Work out the finished part from the listing and answer in its coordinate system (mm). A direction names the side the tool comes from. Round coordinates to 2 decimals unless told otherwise and drop trailing zeros. Loops run counter-clockwise (first coordinate to the right, second up) from the corner with the lowest first, then second, coordinate; pieces in that order, holes last. Notation, with made-up numbers: M 36.25,63 L 44.25,63 A14 cw 44.25,88 Z; hole C 41.5,89.25 d2. An arc over 180 degrees is marked long. One line per item, written item: value.
```python
from build123d import *

# Parameters (mm, degrees)
CROQUIS1_W            = 6
CROQUIS1_H            = 15
CROQUIS2_R            = 4.41619294
CORTAR_EXTRUIR1_DEPTH = 46.572058325


with BuildPart() as part:
    # Croquis1 → Revolución1 (revolve)
    with BuildSketch(Plane.XY):
        with BuildLine():
            Line((7.75, -7.051316702), (7.433772234, -7))
            Line((7.433772234, -7), (3.25, -7))
            Line((3.25, -7), (3.25, 6))
            ThreePointArc((3.25, 6), (4.75, 7.5), (3.25, 9))
            Line((3.25, 9), (1.25, 9))
            Line((1.25, 9), (1.25, -9))
            Line((1.25, -9), (4.765255872, -9))
            Line((4.765255872, -9), (7.75, -9))
            Line((7.75, -9), (7.75, -7.051316702))
        make_face()
        Polygon((7.75, -21), (7.75, -9), (4.765255872, -9), (1.25, -9), (1.25, -21), (7.25, -21), align=None)
        with Locations((4.25, -28.5)):
            Rectangle(CROQUIS1_W, CROQUIS1_H)
    revolve(axis=Axis((-7.75, -7, 0), (0, 1, 0)))

    # Croquis2 → Cortar-Extruir1 (cut, through all)
    with BuildSketch(Plane.XY):
        with Locations((-7.75, -14.025658351)):
            Circle(CROQUIS2_R)
    extrude(amount=-CORTAR_EXTRUIR1_DEPTH, mode=Mode.SUBTRACT)


solid = part.part
```
1) Find the intervals of material crossed by probe 1 along X at (y, z) = (-22, 0); probe 2 along Z at (x, y) = (-7.75, -3); probe 3 along Y at (x, z) = (-7.75, -14), in increasing order. Write a range as from..to.
Check values:
probe 1: -22.75..-16.75, 1.25..7.25
probe 2: -11..-9, 9..11
probe 3: -36..-18.44, -9.61..-7
2) For faces 1 (the face through (-0.598, -13.928, 13.751)), 2 (the face through (-10.13, -0.41, 10.74)), 3 (the face through (-11.005, -11.041, -11.626)), determine the directions among +Z, -Z, +X, -X, +Y, -Y from which every point of the face is accessible in a straight line to the end or side of a thin tool.
Check values:
face 1: +Y, -Y
face 2: none
face 3: -Z
3) Find section A-A (z = 0). Give the vertices of the cut face in (x, y).
Check values:
outline: M -23.25,-21 L -22.75,-21 L -22.75,-36 L -16.75,-36 L -16.75,9 L -18.75,9 A1.5 ccw -18.75,6 L -18.75,-7 L -22.93,-7 L -23.25,-7.05 Z; M 1.25,-36 L 7.25,-36 L 7.25,-21 L 7.75,-21 L 7.75,-7.05 L 7.43,-7 L 3.25,-7 L 3.25,6 A1.5 ccw 3.25,9 L 1.25,9 Z
4) Find section B-B (x = -7.75). Give the vertices of the cut face in (y, z), then the cut area to 3 significant figures.
Check values:
outline: M -36,-15 L -21,-15 L -21,-15.5 L -18.44,-15.5 L -18.44,-9 L -36,-9 Z; M -36,9 L 9,9 L 9,11 A1.5 ccw 6,11 L -7,11 L -7,15.18 L -7.05,15.5 L -21,15.5 L -21,15 L -36,15 Z; M -9.61,-15.5 L -7.05,-15.5 L -7,-15.18 L -7,-11 L 6,-11 A1.5 ccw 9,-11 L 9,-9 L -9.61,-9 Z
area: 376 mm2
5) Each of these flat-tipped pins is pushed along its axis until it touches: pin 1 (5 mm diameter, centred on y = -9, z = 7, fed in from -X); pin 2 (12 mm diameter, centred on x = 4.5, y = -29, fed in from -Z); pin 3 (7 mm diameter, centred on x = -7.75, y = -14.03, fed in from -Z). Where does it stop, or does it pass through?
Check values:
pin 1: x = -22.58
pin 2: z = -13.64
pin 3: z = 8.29
6) Find section C-C (y = 1.5). Give the vertices of the cut face in (x, z).
Check values:
outline: C -7.75,0 d22; hole C -7.75,0 d18
7) Find section D-D (x = -4). Give the number of separate pieces and of enclosed holes in the cut face, then the cut area to 3 significant figures.
Check values:
separate pieces: 3
enclosed holes: 0
area: 427 mm2
8) The mould has two halves that part along Y. Classify faces 4 (the face through (-14.2, -36, 6.5)), 5 (the face through (-18, -7, -5)), 6 (the face through (-22.735, -28.395, -0.66)): +Y half, -Y half, draft (parallel to the pull), parting line (faces both ways), or undercut.
Check values:
face 4: -Y half
face 5: undercut
face 6: draft
